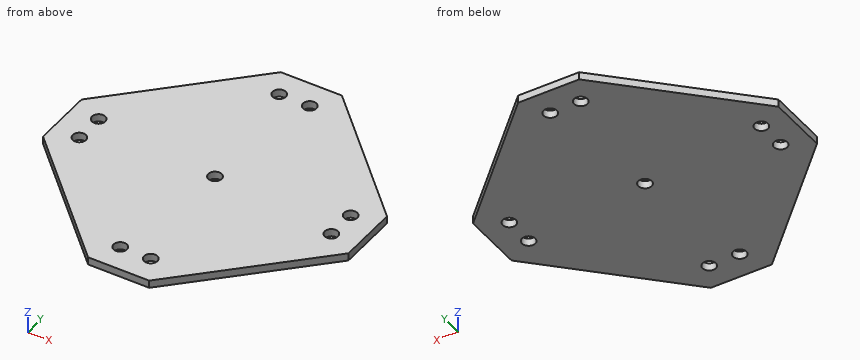
```python
from build123d import *

# Parameters (mm, degrees)
BOSS_EXTRUDE1_DEPTH = 2
CUT_EXTRUDE1_START  = -3
SKETCH2_R           = 1.75
CUT_EXTRUDE1_DEPTH  = 4
CIRPATTERN1_COUNT   = 4


with BuildPart() as part:
    # Sketch1 → Boss-Extrude1 (new body)
    with BuildSketch(Plane.XY):
        Polygon((-8, 40), (8, 40), (40, 8), (40, -8), (8, -40), (-8, -40), (-40, -8), (-40, 8), align=None)
    extrude(amount=BOSS_EXTRUDE1_DEPTH)

    # Sketch2 → Cut-Extrude1 (cut)
    with BuildSketch(Plane.XY.offset(2).offset(CUT_EXTRUDE1_START)):
        with Locations((-4, 33)):
            Circle(SKETCH2_R)
        with Locations((4, 33)):
            Circle(SKETCH2_R)
        Circle(SKETCH2_R)
    cut_extrude1 = extrude(amount=CUT_EXTRUDE1_DEPTH, mode=Mode.SUBTRACT)

    # CirPattern1: Cut-Extrude1 ×4 about axis
    cirpattern1_axis = Axis((0, 0, 0), (0, 0, 1))
    for i in range(1, CIRPATTERN1_COUNT):
        add(cut_extrude1.rotate(cirpattern1_axis, i * 360 / CIRPATTERN1_COUNT), mode=Mode.SUBTRACT)


solid = part.part
```
Here's how the part is built. I have some questions about the finished solid (model axes, mm). Give positions to 0.01 mm unless a question says otherwise; leave off trailing zeros. Loops run counter-clockwise (first coordinate to the right, second up) from the corner with the lowest first, then second, coordinate; pieces in that order, holes last. Notation, with made-up numbers: (59, -14.5) -> (112, -14.5) arc R30 cw to (112, 9.5) -> close; hole circle Ø11 at (-35, -23). An arc over 180 degrees is marked (long way). Use one line per item in the form item = value. Start each with the question number.
1) For P1, Ø10, axis at x = -31.5, y = -28, coming from the -Z side; P2, Ø1, axis at x = 24.5, z = 0.5, coming from the -Y side, each with a flat end and sliding along its axis, tell me the tip position at first contact or that it passes through.
2) Imagine slicing it at C-C (x = -33). Please give me the cut outline in (y, z), then the cut area to 3 significant figures.
3) Imagine slicing it at A-A (x = 0). Please give me the cut outline in (y, z).
4) Imagine slicing it at D-D (z = 0.65). Count the separate pieces of the cut face and the enclosed holes in it, then the cut area to 3 significant figures.
5) Imagine slicing it at B-B (y = -4). Please give me the cut outline in (x, z), then the cut area to 3 significant figures.
6) Please list where these lines run through material, in increasing order: line 1 along Y through (x, z) = (-4, 0.9); line 2 along Y through (x, z) = (-34, 0.9).
Check values:
q1.P1 = through
q1.P2 = -24
q2.outline = (-15, 0) -> (-5.75, 0) -> (-5.75, 2) -> (-15, 2) -> close; (-2.25, 0) -> (2.25, 0) -> (2.25, 2) -> (-2.25, 2) -> close; (5.75, 0) -> (15, 0) -> (15, 2) -> (5.75, 2) -> close
q2.area = 46.0 mm^2
q3.outline = (-40, 0) -> (-1.75, 0) -> (-1.75, 2) -> (-40, 2) -> close; (1.75, 0) -> (40, 0) -> (40, 2) -> (1.75, 2) -> close
q4.separate_pieces = 1
q4.enclosed_holes = 9
q4.area = 4,270 mm^2
q5.outline = (-40, 0) -> (-34.75, 0) -> (-34.75, 2) -> (-40, 2) -> close; (-31.25, 0) -> (31.25, 0) -> (31.25, 2) -> (-31.25, 2) -> close; (34.75, 0) -> (40, 0) -> (40, 2) -> (34.75, 2) -> close
q5.area = 146 mm^2
q6.line_1 = -40 to -34.75, -31.25 to 31.25, 34.75 to 40
q6.line_2 = -14 to -5.44, -2.56 to 2.56, 5.44 to 14
